Verification items for the finished model (mm, model axes). Coordinates: 2 decimals unless noted, no trailing zeros. Order: outer loops, then holes, each group sorted by start corner. A loop starts at its lowest first (then second) coordinate and runs counter-clockwise, first axis right, second up.
Q1. Cross-section at A-A, the plane y = 3.75. Record the boundary of the cut face in (x, z), and give its area (3 significant figures).
Q2. Thickness scan on line 1 (Z direction, x = -1.25, y = 11.75); line 2 (Z direction, x = -0.5, y = 12.5). Record the ranges inside material, lowest first.
Q3. Draft check along Z on faces 1 (the flat face through (0, 0, 0)), 2 (the cylindrical face through (-3.905, 7.003, -0.867)). Enter one of: pulls with the +Z half, pulls with the -Z half, needs draft (parallel to the pull), parting line crosses it, or undercut.
Q4. Depth check by flat-ended pin: P1, Ø1.5, axis at y = 11, z = -2, coming from the -X side; P2, Ø4, axis at x = 1, y = 10.5, coming from the +Z side; P3, Ø1, axis at y = 1.5, z = -1.5, coming from the +X side; P4, Ø1, axis at y = 10.5, z = 3, coming from the +X side. Enter the tip coordinate at first touch or a pass-through.
from build123d import *

# Parameters (mm, degrees)
SKETCH_1_R      = 4
EXTRUDE_1_DEPTH = 15
CHAMFER_1_SIZE  = 1
FILLET_1_R      = 0.2


with BuildPart() as part:
    # 草图1 → 凸台-拉伸1 (new body)
    with BuildSketch(Plane(origin=(0, 0, 0), x_dir=(1, 0, 0), z_dir=(0, 1, 0))):
        with Locations(Location((0, 0, 0), (0, 0, 270))):
            Circle(SKETCH_1_R)
    extrude(amount=EXTRUDE_1_DEPTH)

    # 倒角1
    chamfer_1_edges = [part.edges().sort_by_distance(p)[0] for p in [
        (0, 15, -4),
    ]]
    chamfer(chamfer_1_edges, length=CHAMFER_1_SIZE)

    # 圆角1
    fillet_1_edges = [part.edges().sort_by_distance(p)[0] for p in [
        (0, 0, -4),
    ]]
    fillet(fillet_1_edges, radius=FILLET_1_R)


solid = part.part
Check values:
1. outline: circle Ø8 at (0, 0)
1. area: 50.3 mm2
2. line 1: z = -3.8 to 3.8
2. line 2: z = -3.97 to 3.97
3. face 1: needs draft
3. face 2: parting line crosses it
4. P1: stops at x = -3.8
4. P2: stops at z = 4
4. P3: stops at x = 3.87
4. P4: stops at x = 3.12
